Input: dimensioned drawing with shaded views. Units: mm. Origin: part minimum x, y, z. A direction names the side the tool comes from. Round coordinates to 2 decimals unless told otherwise and drop trailing zeros. Order: outer loops, then holes, each group sorted by start corner. A loop starts at its lowest first (then second) coordinate and runs counter-clockwise, first axis right, second up. Notation, with made-up numbers: M 55,58.5 L 112,58.5 A34 cw 112,93.5 Z; hole C -24,79.25 d1. An arc over 180 degrees is marked long. Use one line per item in the form item = value. Start each with the question number.
Q1. Material intervals for probe 1 along Z at (x, y) = (12, 10.25); probe 2 along Y at (x, z) = (6.75, 12.25), sorted ascending.
Q2. Section D-D (x = 6.5). Return the cut outline in (y, z).
Q3. Section C-C (z = 11). Return the cut outline in (x, y).
Q4. Reachability of the marked faces 1, 2, 3, 4 and 5 from +Z, -Z, +X, -X, +Y, -Y: full face, straight path, thin tool, end or side. Return the list, or none.
Q5. Contact query for flat-ended pins moving along their axis: pin 1 (0.9 mm diameter, centred on y = 6.5, z = 11.5, fed in from -X); pin 2 (0.9 mm diameter, centred on y = 7, z = 2.5, fed in from +X); pin 3 (1 mm diameter, centred on x = 4.5, y = 9, fed in from +Z); pin 4 (2 mm diameter, centred on x = 10.5, z = 2.5, fed in from -Y). Output: stop coordinate, or through.
Q6. Section B-B (x = 3.75). Return the cut outline in (y, z).
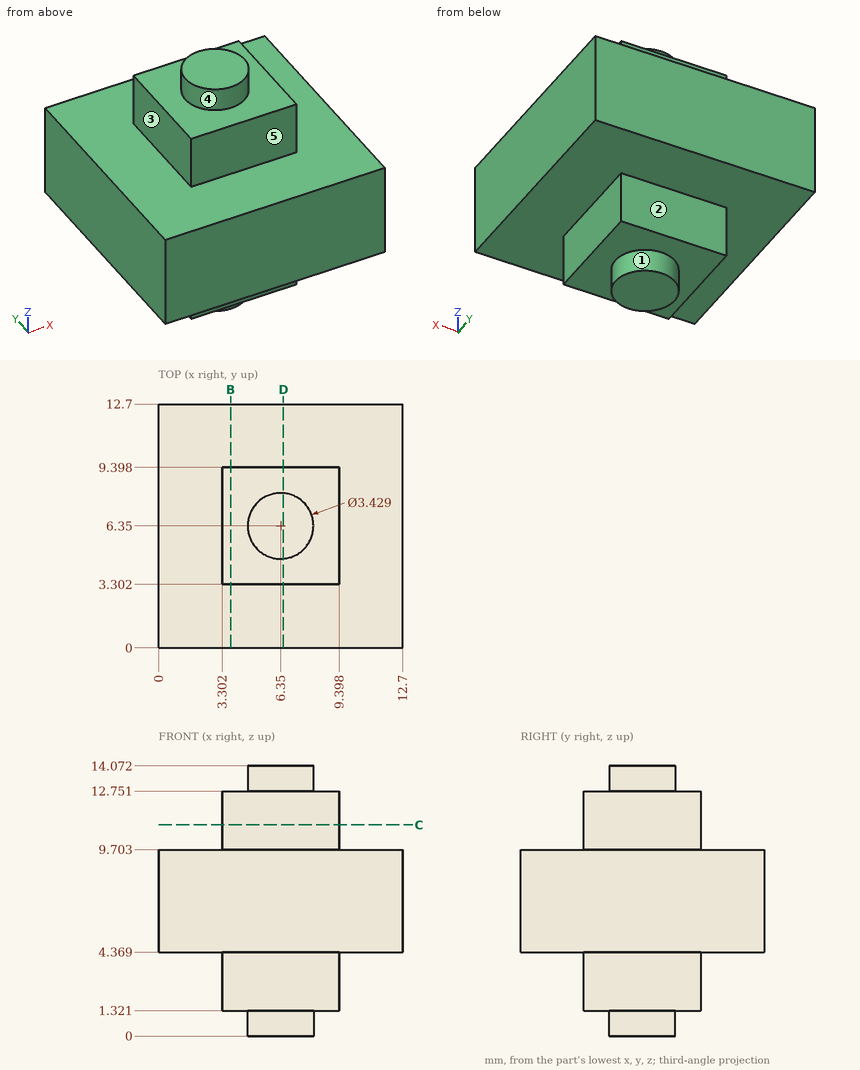
Results list:
q1.probe_1 = 4.37 to 9.7
q1.probe_2 = 3.3 to 9.4
q2.outline = M 0,4.37 L 3.3,4.37 L 3.3,1.32 L 4.64,1.32 L 4.64,0 L 8.06,0 L 8.06,1.32 L 9.4,1.32 L 9.4,4.37 L 12.7,4.37 L 12.7,9.7 L 9.4,9.7 L 9.4,12.75 L 8.06,12.75 L 8.06,14.07 L 4.64,14.07 L 4.64,12.75 L 3.3,12.75 L 3.3,9.7 L 0,9.7 Z
q3.outline = M 3.3,3.3 L 9.4,3.3 L 9.4,9.4 L 3.3,9.4 Z
q4.face_1 = -Z
q4.face_2 = -Z, +X, -X, +Y
q4.face_3 = +Z, -X, +Y, -Y
q4.face_4 = +Z
q4.face_5 = +Z, +X, -X, -Y
q5.pin_1 = 3.3
q5.pin_2 = 9.4
q5.pin_3 = 12.75
q5.pin_4 = through
q6.outline = M 0,4.37 L 3.3,4.37 L 3.3,1.32 L 9.4,1.32 L 9.4,4.37 L 12.7,4.37 L 12.7,9.7 L 9.4,9.7 L 9.4,12.75 L 3.3,12.75 L 3.3,9.7 L 0,9.7 Z
